Here's how the part is built. I have some questions about the finished solid (model axes, mm). Give positions to 0.01 mm unless a question says otherwise; leave off trailing zeros. Write each loop counter-clockwise with the first axis right and the second up, starting at its lowest first coordinate (ties: lowest second). Pieces come first, ordered by that corner, then holes. Notation, with made-up numbers: (75, 69) - (114, 69) arc R12 cw to (114, 91) - close; hole circle Ø8 at (67, -33). An arc over 180 degrees is marked (long way). Write each question's results on one line, items separated by ' | '. Start each with the question number.
Item 1: Suppose I cut it at B-B on z = 3. List the corners of the cut face in (x, y) for me, then the cut area to 3 significant figures.
Item 2: Please list where these lines run through material, in increasing order: line 1 along Y through (x, z) = (166, 1.15); line 2 along Y through (x, z) = (82.5, 2.1); line 3 along X through (y, z) = (-3, 2).
Item 3: Suppose I cut it at D-D on y = -35.85. List the corners of the cut face in (x, z) for me, then the cut area to 4 significant figures.
Item 4: Will these pins go through, and if not, where does the flat tip stop? P1, Ø2.5, axis at x = 55.33, y = -35.85, coming from the +Z side; P2, Ø1.5, axis at y = 5, z = 1.5, coming from the -X side.
Item 5: Suppose I cut it at A-A on x = 148. List the corners of the cut face in (y, z) for me.
Item 6: Suppose I cut it at C-C on x = 166. List the corners of the cut face in (y, z) for me.
Autodesk Inventor part; units mm, degrees
ref_plane "YZ Plane" through (0, 0, 0) normal (1, 0, 0) x (0, 1, 0)
ref_plane "XZ Plane" through (0, 0, 0) normal (0, 1, 0) x (-1, 0, 0)
ref_plane "XY Plane" through (0, 0, 0) normal (0, 0, 1) x (1, 0, 0)
sketch "Boceto1" plane through (0, 0, 0) normal (0, 0, 1) x (1, 0, 0)
  line L0 (0, -32.35) -> (0, -39.35)
  line L1 (0, -39.35) -> (169, -39.35)
  arc A0 (169, -39.35) -> (169.5, -38.85) centre (169, -38.85) ccw
  line L2 (169.5, -38.85) -> (169.5, 38.85)
  arc A1 (169.5, 38.85) -> (169, 39.35) centre (169, 38.85) ccw
  line L3 (169, 39.35) -> (0, 39.35)
  line L4 (0, 39.35) -> (0, 32.35)
  line L5 (0, 32.35) -> (162.5, 32.35)
  line L6 (162.5, 32.35) -> (162.5, -32.35)
  line L7 (162.5, -32.35) -> (0, -32.35)
  circle A2 centre (166, 35.85) radius 2.15
  circle A3 centre (166, -35.85) radius 2.15
  circle A4 centre (55.3333, 35.85) radius 2.15
  circle A5 centre (55.3333, -35.85) radius 2.15
  point P0 (0, 0)
extrude "Extrusión1" add sketch "Boceto1" along normal blind 5
properties part number "ExtensionMarco"
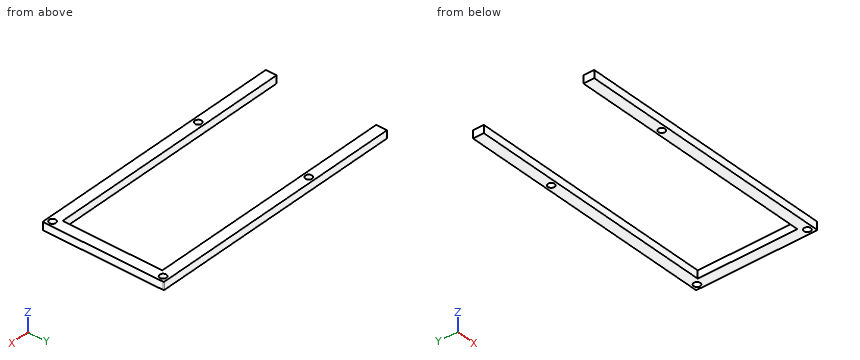
Checked values:
1) outline: (0, -39.35) - (169, -39.35) arc R0.5 ccw to (169.5, -38.85) - (169.5, 38.85) arc R0.5 ccw to (169, 39.35) - (0, 39.35) - (0, 32.35) - (162.5, 32.35) - (162.5, -32.35) - (0, -32.35) - close; hole circle Ø4.3 at (55.33, -35.85); hole circle Ø4.3 at (55.33, 35.85); hole circle Ø4.3 at (166, -35.85); hole circle Ø4.3 at (166, 35.85) | area: 2,770 mm^2
2) line 1: y = -39.35 to -38, -33.7 to 33.7, 38 to 39.35 | line 2: y = -39.35 to -32.35, 32.35 to 39.35 | line 3: x = 162.5 to 169.5
3) outline: (0, 0) - (53.18, 0) - (53.18, 5) - (0, 5) - close; (57.48, 0) - (163.85, 0) - (163.85, 5) - (57.48, 5) - close; (168.15, 0) - (169.5, 0) - (169.5, 5) - (168.15, 5) - close | area: 804.5 mm^2
4) P1: passes through | P2: stops at x = 162.5
5) outline: (-39.35, 0) - (-32.35, 0) - (-32.35, 5) - (-39.35, 5) - close; (32.35, 0) - (39.35, 0) - (39.35, 5) - (32.35, 5) - close
6) outline: (-39.35, 0) - (-38, 0) - (-38, 5) - (-39.35, 5) - close; (-33.7, 0) - (33.7, 0) - (33.7, 5) - (-33.7, 5) - close; (38, 0) - (39.35, 0) - (39.35, 5) - (38, 5) - close
